from build123d import *

# Parameters (mm, degrees)
CYLINDER208_R     = 3.75
CYLINDER208_DEPTH = 10
TUBE006_R         = 16
TUBE006_R_2       = 14.7
TUBE006_DEPTH     = 250


with BuildPart() as cylinder208:
    # Cylinder208 → Cylinder208 (new body)
    with BuildSketch(Plane(origin=(0, -8, -36.5), x_dir=(1, 0, 0), z_dir=(0, -1, 0))):
        Circle(CYLINDER208_R)
    extrude(amount=CYLINDER208_DEPTH)


with BuildPart() as metalholder:
    # Tube006 → Tube006 (new body)
    with BuildSketch(Plane.XY.offset(-277)):
        Circle(TUBE006_R)
        Circle(TUBE006_R_2, mode=Mode.SUBTRACT)
    extrude(amount=TUBE006_DEPTH)

    # Cut150: cut Cylinder208
    add(cylinder208.part, mode=Mode.SUBTRACT)


with BuildPart() as metalholder_1:
    # Cut150 placement: moved
    add(metalholder.part.moved(Location((215, -20, 620))))


solid = metalholder_1.part
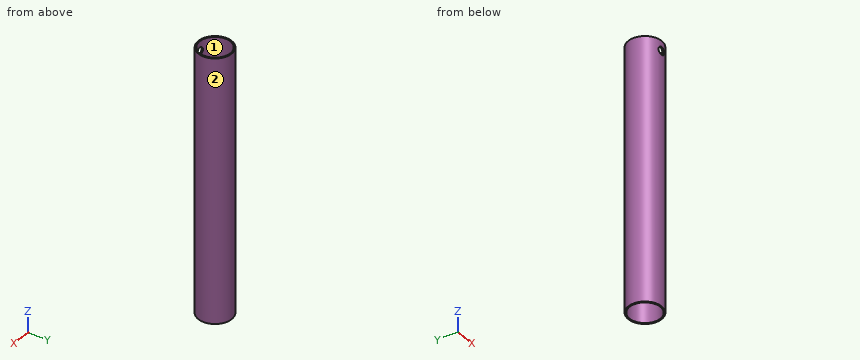
Can you work these out from the model? Positions are in its coordinate system, mm. Face numbers are marked on the shaded views. Round coordinates to 2 decimals unless told otherwise and drop trailing zeros. Loops run counter-clockwise (first coordinate to the right, second up) from the corner with the lowest first, then second, coordinate; pieces in that order, holes last. Notation, with made-up numbers: (-6, 51) - (20, 51) arc R34 ccw to (20, 90) - close; hole circle Ø10 at (-36.5, -34). An arc over 180 degrees is marked (long way). Write item = value, one per line. Start each with the question number.
(1) If I drill on probe 1 along Y at (x, z) = (215.5, 522); probe 2 along Z at (x, y) = (215, -35.2); probe 3 along X at (y, z) = (-20.5, 571), over which ranges is the centre line in solid material (lowest first)? Write a range as [from, to].
(2) If we section it at D-D (z = 583.5): Please give me the cut outline in (x, y), and give its area (3 significant figures).
(3) If we section it at C-C (z = 364.5): Please give me the cut outline in (x, y), and give its area (3 significant figures).
(4) If we section it at B-B (x = 208): Please give me the cut outline in (y, z).
(5) If we mould it in two halves opening along X, with no side actions, what happens to the marked faces 1 and 2? For each: released by +X, released by -X, zero draft, split by the parting line, or undercut.
(6) For P1, Ø5, axis at x = 208.5, z = 408.5, coming from the +Y side; P2, Ø10, axis at x = 215, z = 583.5, coming from the -Y side; P3, Ø4, axis at y = -29, z = 430, coming from the -X side; P4, Ø5, axis at y = -11, z = 495.5, coming from the +X side, each with a flat end and sliding along its axis, tell me the tip position at first contact or that it passes through.
(7) If we section it at A-A (y = -20): Please give me the cut outline in (x, z), and give its area (3 significant figures).
Ans:
q1.probe_1 = [-35.99, -34.69], [-5.31, -4.01]
q1.probe_2 = [343, 579.75], [587.25, 593]
q1.probe_3 = [199.01, 200.31], [229.69, 230.99]
q2.outline = (211.25, -35.55) - (211.25, -34.21) arc R14.7 cw (long way) to (218.75, -34.21) - (218.75, -35.55) arc R16 ccw (long way) to start
q2.area = 116 mm²
q3.outline = circle Ø32 at (215, -20); hole circle Ø29.4 at (215, -20)
q3.area = 125 mm²
q4.outline = (-34.39, 343) - (-32.93, 343) - (-32.93, 593) - (-34.39, 593) - close; (-7.07, 343) - (-5.61, 343) - (-5.61, 593) - (-7.07, 593) - close
q5.face_1 = undercut
q5.face_2 = split by the parting line
q6.P1 = -4.51
q6.P2 = -36
q6.P3 = 200.61
q6.P4 = 229.62
q7.outline = (199, 343) - (200.3, 343) - (200.3, 593) - (199, 593) - close; (229.7, 343) - (231, 343) - (231, 593) - (229.7, 593) - close
q7.area = 650 mm²
